```python
from build123d import *

# Parameters (mm, degrees)
CI_DEPTH                   = 7.5
CI_DEPTH_BACK              = 7.5
SKETCHCI_M_STRSKETCHNAME_W = 21.04999997
SKETCHCI_M_STRSKETCHNAME_H = 194.778741597
CUT_EXTRUDE_522_DEPTH      = 7.5
PATTERN_LINEAR_579_COUNT   = 31
PATTERN_LINEAR_579_PITCH   = 6.283185307
EXTRUDE3_DEPTH             = 194.164953792
EXTRUDE3_DEPTH_BACK        = 194.164953792


with BuildPart() as part:
    # SketchCI.m_strSketchName → 拉伸CI (new, two sides: drawn at the far end of the back side and taken through both)
    with BuildSketch(Plane.XY.offset(-CI_DEPTH_BACK)):
        with Locations((8.525000015, -94.247778193)):
            Rectangle(SKETCHCI_M_STRSKETCHNAME_W, SKETCHCI_M_STRSKETCHNAME_H)
    extrude(amount=CI_DEPTH + CI_DEPTH_BACK)

    # Sketch 415 → Cut-Extrude 522 (cut, symmetric)
    with BuildSketch(Plane.XY):
        with BuildLine():
            Line((-1.99999997, 2.298736761), (-1.99999997, -2.298736761))
            Line((-1.99999997, -2.298736761), (2.105212054, -0.804561779))
            ThreePointArc((2.105212054, -0.804561779), (2.391491191, -0.584892071), (2.499999962, -0.240746215))
            Line((2.499999962, -0.240746215), (2.499999962, 0.240746215))
            ThreePointArc((2.499999962, 0.240746215), (2.391491191, 0.584892071), (2.105212054, 0.804561779))
            Line((2.105212054, 0.804561779), (-1.99999997, 2.298736761))
        make_face()
    cut_extrude_522 = extrude(amount=CUT_EXTRUDE_522_DEPTH, both=True, mode=Mode.SUBTRACT)

    # Pattern Linear 579: Cut-Extrude 522 ×31
    with Locations(*[(0, -i * PATTERN_LINEAR_579_PITCH, 0) for i in range(1, PATTERN_LINEAR_579_COUNT)]):
        add(cut_extrude_522, mode=Mode.SUBTRACT)

    # Sketch4 → Extrude3 (cut, two sides: drawn at the far end of the back side and taken through both)
    with BuildSketch(Plane.XY.offset(7.5).offset(-EXTRUDE3_DEPTH_BACK)):
        Polygon((328.075571379, -141.637148991), (19.05, -141.637148991), (-18.275447969, -141.637148991), (-327.301019347, -141.637148991), (-327.301019347, 476.413993766), (328.075571379, 476.413993766), align=None)
    extrude(amount=EXTRUDE3_DEPTH + EXTRUDE3_DEPTH_BACK, mode=Mode.SUBTRACT)


solid = part.part
```
The model under review builds one solid part; all positions refer to its coordinate system, in mm. A direction names the side the tool comes from. Coordinates: 2 decimals unless noted, no trailing zeros. Write each loop counter-clockwise with the first axis right and the second up, starting at its lowest first coordinate (ties: lowest second). Pieces come first, ordered by that corner, then holes. Notation, with made-up numbers: (16.25, 35.5) - (55.25, 35.5) arc R24 ccw to (55.25, 73.5) - close; hole circle Ø3 at (45.5, 45.25). An arc over 180 degrees is marked (long way). Write item = value, one per line.
(1) Machinability: for faces 4 (the face through (8, -166, 7.5)), 5 (the face through (0.02, -152.36, 0.11)), which of the approach directions +Z, -Z, +X, -X, +Y, -Y give a long, thin tool a straight path to every point of the face, cutting with its end or side? Answer none if there is none.
Result sheet:
face_4 = +Z, +X, -X, +Y, -Y
face_5 = +Z, -Z, -X
(2) For line 1 (X direction, y = -176, z = 1.25); line 2 (X direction, y = -145, z = -4.25), list the stretches that pass through material, from the lowest coordinate up. Write a range as [from, to].
Result sheet:
line_1 = [2.5, 19.05]
line_2 = [2.45, 19.05]
(3) Mouldability with a two-part tool opening along Y and no side actions: class faces 1 (the face through (8, -141.637, 0)), 2 (the face through (19.05, -167, 0)), 3 (the face through (0.08, -180.67, 0.11)) as pulls with the +Y half, pulls with the -Y half, needs draft (parallel to the pull), parting line crosses it, or undercut.
Result sheet:
face_1 = pulls with the +Y half
face_2 = needs draft
face_3 = undercut
(4) Consider section A-A, the plane x = 1.25. State how many separate pieces and enclosed holes the cut face has, then the cut area to 3 significant figures.
Result sheet:
separate_pieces = 9
enclosed_holes = 0
area = 482 mm^2
(5) For P1, Ø0.5, axis at y = -188.5, z = -0.5, coming from the -X side, flat-tipped, find the tip position at first contact; note if it passes through.
Result sheet:
P1 = 2.5
(6) Consider section B-B, the plane y = -155.5. Give the boundary of the cut face in (x, z).
Result sheet:
outline = (-0.02, -7.5) - (19.05, -7.5) - (19.05, 7.5) - (-0.02, 7.5) - close
